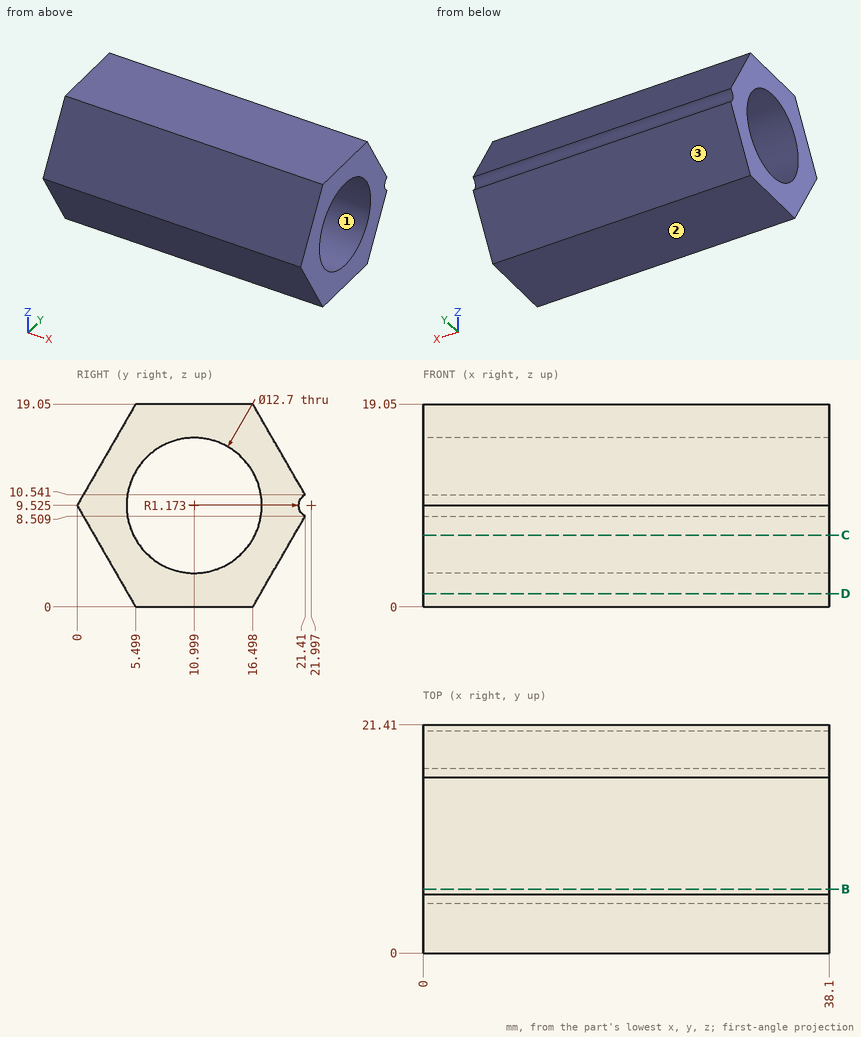
For this review, use the dimensioned drawing (mm, ordinates from the lowest corner) and the shaded views. Coordinates: 2 decimals unless noted, no trailing zeros. Loops run counter-clockwise (first coordinate to the right, second up) from the corner with the lowest first, then second, coordinate; pieces in that order, holes last.
1. Mouldability with a two-part tool opening along Y and no side actions: class the marked faces 1, 2 and 3 as +Y half, -Y half, draft (parallel to the pull), parting line (faces both ways), or undercut.
2. Insertion check: P1, Ø8, axis at x = 12.5, z = 11, coming from the -Y side; P2, Ø1, axis at x = 29, z = 3.5, coming from the -Y side; P3, Ø1.5, axis at x = 26.5, y = 2.5, coming from the -Z side (1 decimal). Each pin has a flat end and moves straight along its axis. Give the tip position at first contact, or say it passes through.
3. Add section B-B, the plane y = 6. Give the boundary of the cut face in (x, z).
4. Add section C-C, the plane z = 6.75. Give the boundary of the cut face in (x, y) (1 decimal).
5. Add section D-D, the plane z = 1.25. Give the boundary of the cut face in (x, y), then the cut area to 3 significant figures.
6. For line 1 (Y direction, x = 8, z = 8) (1 decimal); line 2 (Y direction, x = 16, z = 4.75) (1 decimal); line 3 (Z direction, x = 28.5, y = 12.75), list the stretches that pass through material, from the lowest coordinate up.
Result:
1. face 1: undercut
1. face 2: draft
1. face 3: +Y half
2. P1: stops at y = 0
2. P2: stops at y = 3.19
2. P3: stops at z = 3.9
3. outline: (0, 0) - (38.1, 0) - (38.1, 5.61) - (0, 5.61) - close; (0, 13.44) - (38.1, 13.44) - (38.1, 19.05) - (0, 19.05) - close
4. outline: (0, 1.6) - (38.1, 1.6) - (38.1, 5.3) - (0, 5.3) - close; (0, 16.7) - (38.1, 16.7) - (38.1, 20.4) - (0, 20.4) - close
5. outline: (0, 4.78) - (38.1, 4.78) - (38.1, 17.22) - (0, 17.22) - close
5. area: 474 mm2
6. line 1: y = 0.9 to 4.8, 17.2 to 21.1
6. line 2: y = 2.8 to 6.8, 15.2 to 19.2
6. line 3: z = 0 to 3.42, 15.63 to 19.05
